```python
from build123d import *

# Parameters (mm, degrees)
SKETCH1_R           = 1.5875
SKETCH1_R_2         = 0.5
BOSS_EXTRUDE1_DEPTH = 1.5875


with BuildPart() as part:
    # Sketch1 → Boss-Extrude1 (new body)
    with BuildSketch(Plane.XY):
        with BuildLine():
            Line((-11.379865944, 21.982845747), (-5.412817802, 24.154673658))
            Line((-5.412817802, 24.154673658), (1.102665928, 6.253529232))
            ThreePointArc((1.102665928, 6.253529232), (5.134627331, 3.736054359), (6.289441106, -0.874888889))
            ThreePointArc((6.289441106, -0.874888889), (6.476937503, -1.505418725), (7.075621245, -1.778))
            Line((7.075621245, -1.778), (8.036200346, -1.778))
            ThreePointArc((8.036200346, -1.778), (8.562245058, -1.578653923), (8.824063125, -1.080745098))
            ThreePointArc((8.824063125, -1.080745098), (8.886673646, -0.243169696), (8.869960358, 0.596576276))
            ThreePointArc((8.869960358, 0.596576276), (9.082128579, 1.191948731), (9.661921104, 1.443592015))
            Line((9.661921104, 1.443592015), (10.93445675, 1.443592015))
            ThreePointArc((10.93445675, 1.443592015), (11.478819393, 1.227516989), (11.726808688, 0.696932016))
            ThreePointArc((11.726808688, 0.696932016), (11.575475742, -2.003027106), (10.810769922, -4.596847826))
            ThreePointArc((10.810769922, -4.596847826), (10.51820634, -4.948283265), (10.080312495, -5.08))
            Line((10.080312495, -5.08), (-3.53553037, -5.08))
            ThreePointArc((-3.53553037, -5.08), (-3.803866846, -5.033267134), (-4.040606138, -4.898571429))
            ThreePointArc((-4.040606138, -4.898571429), (-6.323450723, -0.58006116), (-4.864382214, 4.081701322))
            Line((-4.864382214, 4.081701322), (-11.379865944, 21.982845747))
        make_face()
        Circle(SKETCH1_R, mode=Mode.SUBTRACT)
        with Locations((-7.527610709, 20.681940446)):
            Circle(SKETCH1_R_2, mode=Mode.SUBTRACT)
        with Locations((-6.658879545, 18.295121189)):
            Circle(SKETCH1_R_2, mode=Mode.SUBTRACT)
        with Locations((-5.790148381, 15.908301932)):
            Circle(SKETCH1_R_2, mode=Mode.SUBTRACT)
        with Locations((-4.921417217, 13.521482675)):
            Circle(SKETCH1_R_2, mode=Mode.SUBTRACT)
    extrude(amount=BOSS_EXTRUDE1_DEPTH)


solid = part.part
```
Check sheet for the modelled part. Datum: model origin and axes. Units: mm. A direction names the side the tool comes from. Round coordinates to 2 decimals unless told otherwise and drop trailing zeros. Write each loop counter-clockwise with the first axis right and the second up, starting at its lowest first coordinate (ties: lowest second). Pieces come first, ordered by that corner, then holes. Notation, with made-up numbers: M 68.5,-23 L 104.5,-23 A15 cw 104.5,-15 Z; hole C 55.5,65.5 d10. An arc over 180 degrees is marked long. Write item = value, one per line. Start each with the question number.
1. Section check C-C, the plane x = 0. Record the cut outline in (y, z).
2. Section check A-A, the plane y = 0. Record the cut outline in (x, z), then the cut area to 3 significant figures.
3. Tool access check on faces 1 (the flat face through (-8.077, 12.907, 0.783)), 2 (the cylindrical face through (8.886, -0.255, 0.783)), 3 (the flat face through (10, 1.444, 1)). Record the directions out of +Z, -Z, +X, -X, +Y, -Y that give a thin tool (end or side, any length) a straight path to the whole face; none if there is none.
4. Section check D-D, the plane y = 12.5. Record the cut outline in (x, z), then the cut area to 3 significant figures.
5. Scan lines: line 1 (X direction, y = 1, z = 0.6); line 2 (X direction, y = 21, z = 0.65); line 3 (X direction, y = 18.25, z = 0.1). Record each from-to range of solid material in increasing order. Write a range as [from, to].
6. Section check B-B, the plane z = 1.25. State how many separate pieces and enclosed holes the cut face has, then the cut area to 3 significant figures.
7. Release check for a two-part mould opening along Y. For faces 4 (the flat face through (-2, 6, 1.588)), 5 (the flat face through (-8.438, 23.054, 0.783)), 6 (the cylindrical face through (6.47, -1.5, 0.78)), 7 (the flat face through (3, -5.08, 1)) record: pulls with the +Y half, pulls with the -Y half, needs draft (parallel to the pull), parting line crosses it, or undercut.
Results found:
q1.outline = M -5.08,0 L -1.59,0 L -1.59,1.59 L -5.08,1.59 Z; M 1.59,0 L 9.28,0 L 9.28,1.59 L 1.59,1.59 Z
q2.outline = M -6.35,0 L -1.59,0 L -1.59,1.59 L -6.35,1.59 Z; M 1.59,0 L 6.35,0 L 6.35,1.59 L 1.59,1.59 Z; M 8.89,0 L 11.75,0 L 11.75,1.59 L 8.89,1.59 Z
q2.area = 19.7 mm^2
q3.face_1 = +Z, -Z, -X
q3.face_2 = +Z, -Z
q3.face_3 = +Z, -Z, +X, +Y
q4.outline = M -7.93,0 L -1.17,0 L -1.17,1.59 L -7.93,1.59 Z
q4.area = 10.7 mm^2
q5.line_1 = [-6.27, -1.23], [1.23, 6.27], [8.95, 11.65]
q5.line_2 = [-11.02, -7.91], [-7.14, -4.26]
q5.line_3 = [-10.02, -7.16], [-6.16, -3.26]
q6.separate_pieces = 1
q6.enclosed_holes = 5
q6.area = 255 mm^2
q7.face_4 = needs draft
q7.face_5 = pulls with the +Y half
q7.face_6 = undercut
q7.face_7 = pulls with the -Y half
